For this review, take the finished solid that the model builds, in its own axes (mm). Face numbers are marked on the shaded views. A direction names the side the tool comes from. Round coordinates to 2 decimals unless told otherwise and drop trailing zeros. Loops run counter-clockwise (first coordinate to the right, second up) from the corner with the lowest first, then second, coordinate; pieces in that order, holes last. Notation, with made-up numbers: M -39.5,-33 L -2.5,-33 A21 cw -2.5,-4 Z; hole C -6,5 d8. An arc over 180 degrees is marked long. Write item = value, one per line. Start each with the question number.
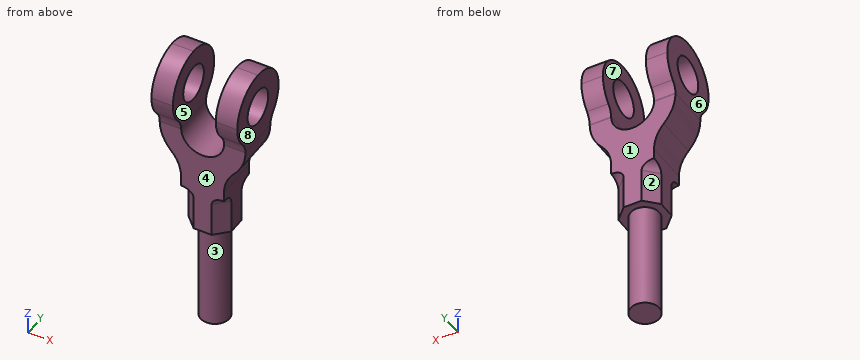
```python
from build123d import *

# Parameters (mm, degrees)
SKETCH1_W           = 120
SKETCH1_H           = 250
BOSS_EXTRUDE1_DEPTH = 100
CUT_EXTRUDE1_DEPTH  = 295.78805946
CUT_EXTRUDE2_DEPTH  = 295.78805946
SKETCH5_R           = 25
CUT_EXTRUDE3_DEPTH  = 295.7880595
CUT_EXTRUDE5_DEPTH  = 60
CUT_EXTRUDE6_DEPTH  = 60
CUT_EXTRUDE7_DEPTH  = 60
CUT_EXTRUDE8_DEPTH  = 60
SKETCH10_R          = 20.176522507
BOSS_EXTRUDE2_DEPTH = 150.7
FILLET1_R           = 12
FILLET2_R           = 12
FILLET3_R           = 12
FILLET4_R           = 12


with BuildPart() as part:
    # Sketch1 → Boss-Extrude1 (new body)
    with BuildSketch(Plane(origin=(0, 0, 0), x_dir=(1, 0, 0), z_dir=(0, 1, 0))):
        with Locations((60, -125)):
            Rectangle(SKETCH1_W, SKETCH1_H)
    extrude(amount=BOSS_EXTRUDE1_DEPTH)

    # Sketch2 → Cut-Extrude1 (cut, through all)
    with BuildSketch(Plane(origin=(0, 100, 0), x_dir=(1, 0, 0), z_dir=(0, 1, 0))):
        with BuildLine():
            ThreePointArc((90, -150), (60, -120), (30, -150))
            Line((30, -150), (30, -250))
            Line((30, -250), (90, -250))
            Line((90, -250), (90, -150))
        make_face()
        with BuildLine():
            Line((120, 0), (90, 0))
            Line((90, 0), (90, -74.501655647))
            ThreePointArc((90, -74.501655647), (93.533981136, -92.965379294), (103.636363636, -108.819084899))
            ThreePointArc((103.636363636, -108.819084899), (115.759222637, -127.843531624), (120, -150))
            Line((120, -150), (120, 0))
        make_face()
        with BuildLine():
            Line((30, -74.501655647), (30, 0))
            Line((30, 0), (0, 0))
            Line((0, 0), (0, -150.000000078))
            ThreePointArc((0, -150.000000078), (4.240777349, -127.84353166), (16.363636364, -108.819084899))
            ThreePointArc((16.363636364, -108.819084899), (26.466018864, -92.965379294), (30, -74.501655647))
        make_face()
    extrude(amount=-CUT_EXTRUDE1_DEPTH, mode=Mode.SUBTRACT)

    # Sketch4 → Cut-Extrude2 (cut, through all)
    with BuildSketch(Plane(origin=(120, 0, 0), x_dir=(0, 0, -1), z_dir=(1, 0, 0))):
        with BuildLine():
            ThreePointArc((-250, 50), (-235.355339059, 85.355339059), (-200, 100))
            Line((-200, 100), (-250, 100))
            Line((-250, 100), (-250, 50))
        make_face()
        with BuildLine():
            Line((-150, 100), (-200, 100))
            ThreePointArc((-200, 100), (-181.742581416, 96.547466813), (-166.006536576, 86.666666667))
            ThreePointArc((-166.006536576, 86.666666667), (-158.59772436, 81.911652295), (-150, 80.019617425))
            Line((-150, 80.019617425), (-150, 100))
        make_face()
        with BuildLine():
            Line((-108.819084899, 100), (-150, 100))
            Line((-150, 100), (-150, 80.019617425))
            ThreePointArc((-150, 80.019617425), (-149.504999586, 80.004904837), (-149.009804864, 80))
            Line((-149.009804864, 80), (0, 80))
            Line((0, 80), (0, 100))
            Line((0, 100), (-74.501655647, 100))
            Line((-74.501655647, 100), (-108.819084899, 100))
        make_face()
        with BuildLine():
            ThreePointArc((-200, 0), (-235.355339059, 14.644660941), (-250, 50))
            Line((-250, 50), (-250, 0))
            Line((-250, 0), (-200, 0))
        make_face()
        with BuildLine():
            ThreePointArc((-166.006536576, 13.333333333), (-181.742581416, 3.452533187), (-200, 0))
            Line((-200, 0), (-150, 0))
            Line((-150, 0), (-150, 19.980382575))
            ThreePointArc((-150, 19.980382575), (-158.59772436, 18.088347705), (-166.006536576, 13.333333333))
        make_face()
        with BuildLine():
            ThreePointArc((-149.009804864, 20), (-149.504999586, 19.995095163), (-150, 19.980382575))
            Line((-150, 19.980382575), (-150, 0))
            Line((-150, 0), (-108.819084899, 0))
            Line((-108.819084899, 0), (-74.501655647, 0))
            Line((-74.501655647, 0), (0, 0))
            Line((0, 0), (0, 20))
            Line((0, 20), (-149.009804864, 20))
        make_face()
    extrude(amount=-CUT_EXTRUDE2_DEPTH, mode=Mode.SUBTRACT)

    # Sketch5 → Cut-Extrude3 (cut, through all)
    with BuildSketch(Plane(origin=(120, 0, 0), x_dir=(0, 0, -1), z_dir=(1, 0, 0))):
        with Locations((-200, 50)):
            Circle(SKETCH5_R)
    extrude(amount=-CUT_EXTRUDE3_DEPTH, mode=Mode.SUBTRACT)

    # Sketch6 → Cut-Extrude5 (cut)
    with BuildSketch(Plane(origin=(0, 0, 0), x_dir=(-1, 0, 0), z_dir=(0, 0, -1))):
        Polygon((-30, 62.6), (-30, 80), (-47.4, 80), align=None)
    extrude(amount=-CUT_EXTRUDE5_DEPTH, mode=Mode.SUBTRACT)

    # Sketch7 → Cut-Extrude6 (cut)
    with BuildSketch(Plane(origin=(0, 0, 0), x_dir=(-1, 0, 0), z_dir=(0, 0, -1))):
        Polygon((-72.6, 80), (-90, 80), (-90, 62.6), align=None)
    extrude(amount=-CUT_EXTRUDE6_DEPTH, mode=Mode.SUBTRACT)

    # Sketch8 → Cut-Extrude7 (cut)
    with BuildSketch(Plane(origin=(0, 0, 0), x_dir=(-1, 0, 0), z_dir=(0, 0, -1))):
        Polygon((-90, 37.4), (-90, 20), (-72.6, 20), align=None)
    extrude(amount=-CUT_EXTRUDE7_DEPTH, mode=Mode.SUBTRACT)

    # Sketch9 → Cut-Extrude8 (cut)
    with BuildSketch(Plane(origin=(0, 0, 0), x_dir=(-1, 0, 0), z_dir=(0, 0, -1))):
        Polygon((-30, 37.4), (-30, 20), (-47.4, 20), align=None)
    extrude(amount=-CUT_EXTRUDE8_DEPTH, mode=Mode.SUBTRACT)

    # Sketch10 → Boss-Extrude2 (add)
    with BuildSketch(Plane(origin=(0, 0, 0), x_dir=(-1, 0, 0), z_dir=(0, 0, -1))):
        with Locations((-60, 50)):
            Circle(SKETCH10_R)
    extrude(amount=BOSS_EXTRUDE2_DEPTH)

    # Fillet1
    fillet1_edges = [part.edges().sort_by_distance(p)[0] for p in [
        (81.3, 28.7, 60),
    ]]
    fillet(fillet1_edges, radius=FILLET1_R)

    # Fillet2
    fillet2_edges = [part.edges().sort_by_distance(p)[0] for p in [
        (81.3, 71.3, 60),
    ]]
    fillet(fillet2_edges, radius=FILLET2_R)

    # Fillet3
    fillet3_edges = [part.edges().sort_by_distance(p)[0] for p in [
        (38.7, 71.3, 60),
    ]]
    fillet(fillet3_edges, radius=FILLET3_R)

    # Fillet4
    fillet4_edges = [part.edges().sort_by_distance(p)[0] for p in [
        (38.7, 28.7, 60),
    ]]
    fillet(fillet4_edges, radius=FILLET4_R)


solid = part.part
```
(1) Add section B-B on z = 40.5. Write out the cut boundary in (x, y), and give its area (3 significant figures).
(2) Draft analysis for pull direction X (two halves, no side actions). For the marked faces 6, 7 and 8, state which applies: +X half, -X half, draft (parallel to the pull), parting line (faces both ways), or undercut.
(3) Wall thickness on L1, parallel to X at y = 47.5, z = 174; L2, parallel to Y at x = 20, z = 200; L3, parallel to X at y = 48.5, z = -113: over which ranges is each line inside the solid? List them lowest first.
(4) Add section A-A on x = 60. Write out the cut boundary in (y, z).
(5) Add section D-D on z = 87. Write out the cut boundary in (x, y).
(6) Tool access review of the marked faces 1, 2, 3, 4 and 5: name each direction out of +Z, -Z, +X, -X, +Y, -Y from which nothing blocks a thin tool from reaching the whole face with its end or side.
(7) For pin 1 Ø4 at (y, z) = (28, 66) entering from -X; pin 2 Ø12 at (x, y) = (88, 51.5) entering from -Z; pin 3 Ø3 at (x, y) = (94, 90) entering from +Z, all flat-tipped, find the tip position at first contact; note any pin that passes through.
(8) Add section C-C on z = -103. Write out the cut boundary in (x, y), and give its area (3 significant figures).
Answer sheet:
q1.outline = M 30,37.4 L 47.4,20 L 72.6,20 L 90,37.4 L 90,62.6 L 72.6,80 L 47.4,80 L 30,62.6 Z
q1.area = 2,990 mm²
q2.face_6 = -X half
q2.face_7 = undercut
q2.face_8 = +X half
q3.L1 = 0 to 30, 90 to 120
q3.L2 = 0 to 25, 75 to 100
q3.L3 = 39.88 to 80.12
q4.outline = M 20,0 L 29.82,0 L 29.82,-150.7 L 70.18,-150.7 L 70.18,0 L 80,0 L 80,120 L 20,120 Z
q5.outline = M 28.41,20 L 91.59,20 L 91.59,80 L 28.41,80 Z
q6.face_1 = -Z, +X, -X, +Y
q6.face_2 = -Z, -X, +Y
q6.face_3 = -Z
q6.face_4 = -Z, +X, -X, -Y
q6.face_5 = +Z, +Y, -Y
q7.pin_1 = 30
q7.pin_2 = 0
q7.pin_3 = 231.9
q8.outline = C 60,50 d40.35
q8.area = 1,280 mm²
